```python
from build123d import *

# Parameters (mm, degrees)
SKETCH1_W           = 10
SKETCH1_H           = 20
SKETCH1_W_2         = 8
SKETCH1_H_2         = 18
BOSS_EXTRUDE1_DEPTH = 300
CUT_EXTRUDE1_REACH  = 302.333
SKETCH2_R           = 2


with BuildPart() as part:
    # Sketch1 → Boss-Extrude1 (new body)
    with BuildSketch(Plane.XY):
        Rectangle(SKETCH1_W, SKETCH1_H)
        Rectangle(SKETCH1_W_2, SKETCH1_H_2, mode=Mode.SUBTRACT)
    extrude(amount=BOSS_EXTRUDE1_DEPTH)

    # Sketch2 → Cut-Extrude1 (cut, up to next)
    with BuildSketch(Plane(origin=(5, 0, 0), x_dir=(0, 0, -1), z_dir=(1, 0, 0)), mode=Mode.PRIVATE) as cut_extrude1_sk1:
        with Locations((-6, 0)):
            Circle(SKETCH2_R)
    cut_extrude1_tool1 = extrude(cut_extrude1_sk1.sketch, amount=-CUT_EXTRUDE1_REACH, mode=Mode.PRIVATE) & part.part
    # Sketch2 → Cut-Extrude1 (cut, up to next)
    with BuildSketch(Plane(origin=(5, 0, 0), x_dir=(0, 0, -1), z_dir=(1, 0, 0)), mode=Mode.PRIVATE) as cut_extrude1_sk2:
        with Locations((-24, 0)):
            Circle(SKETCH2_R)
    cut_extrude1_tool2 = extrude(cut_extrude1_sk2.sketch, amount=-CUT_EXTRUDE1_REACH, mode=Mode.PRIVATE) & part.part
    # Sketch2 → Cut-Extrude1 (cut, up to next)
    with BuildSketch(Plane(origin=(5, 0, 0), x_dir=(0, 0, -1), z_dir=(1, 0, 0)), mode=Mode.PRIVATE) as cut_extrude1_sk3:
        with Locations((-42, 0)):
            Circle(SKETCH2_R)
    cut_extrude1_tool3 = extrude(cut_extrude1_sk3.sketch, amount=-CUT_EXTRUDE1_REACH, mode=Mode.PRIVATE) & part.part
    add(cut_extrude1_tool1.solids().sort_by_distance((5, 0, 6))[0], mode=Mode.SUBTRACT)
    add(cut_extrude1_tool2.solids().sort_by_distance((5, 0, 24))[0], mode=Mode.SUBTRACT)
    add(cut_extrude1_tool3.solids().sort_by_distance((5, 0, 42))[0], mode=Mode.SUBTRACT)


solid = part.part
```
Design review of the part built by this model. Coordinates are the model's own, in mm. A direction names the side the tool comes from. Coordinates: 2 decimals unless noted, no trailing zeros. Order: outer loops, then holes, each group sorted by start corner. A loop starts at its lowest first (then second) coordinate and runs counter-clockwise, first axis right, second up.
1) For faces 1 (the flat face through (5, 0, 148)), 2 (the flat face through (0, 9, 148)), list the 3-axis set-ups (+Z, -Z, +X, -X, +Y, -Y) from which the entire face can be reached by the end or side of a thin tool; tool diameter is ignored.
2) Take a section at A-A, the plane x = -0.25. Give the boundary of the cut face in (y, z), and give its area (3 significant figures).
3) Wall thickness on line 1 along Y through (x, z) = (0, 132); line 2 along X through (y, z) = (-7.5, 22); line 3 along Y through (x, z) = (4.7, 24): over which ranges is each line inside the solid? List them lowest first.
4) Take a section at C-C, the plane z = 80.5. Give the boundary of the cut face in (x, y).
5) Mouldability with a two-part tool opening along Y and no side actions: class faces 3 (the flat face through (0, -10, 148)), 4 (the flat face through (-4.5, 0.8, 0)), 5 (the flat face through (0, -9, 148)) as +Y half, -Y half, draft (parallel to the pull), parting line (faces both ways), or undercut.
6) Take a section at B-B, the plane y = 5. Give the boundary of the cut face in (x, z).
Returned:
1. face 1: +Z, -Z, +X, +Y, -Y
1. face 2: +Z, -Z
2. outline: (-10, 0) - (-9, 0) - (-9, 300) - (-10, 300) - close; (9, 0) - (10, 0) - (10, 300) - (9, 300) - close
2. area: 600 mm2
3. line 1: y = -10 to -9, 9 to 10
3. line 2: x = -5 to -4, 4 to 5
3. line 3: y = -10 to -2, 2 to 10
4. outline: (-5, -10) - (5, -10) - (5, 10) - (-5, 10) - close; hole (-4, -9) - (4, -9) - (4, 9) - (-4, 9) - close
5. face 3: -Y half
5. face 4: draft
5. face 5: undercut
6. outline: (-5, 0) - (-4, 0) - (-4, 300) - (-5, 300) - close; (4, 0) - (5, 0) - (5, 300) - (4, 300) - close
